Build history of the part. All positions in model axes, mm. Face numbers are marked on the shaded views. A direction names the side the tool comes from. Coordinates: 2 decimals unless noted, no trailing zeros. Order: outer loops, then holes, each group sorted by start corner. A loop starts at its lowest first (then second) coordinate and runs counter-clockwise, first axis right, second up. Notation, with made-up numbers: M -12.5,6.25 L 2.5,6.25 A19 ccw 2.5,30.25 Z; hole C 37,-18.5 d3. An arc over 180 degrees is marked long. Use a Markdown table: item, result. Add a question column.
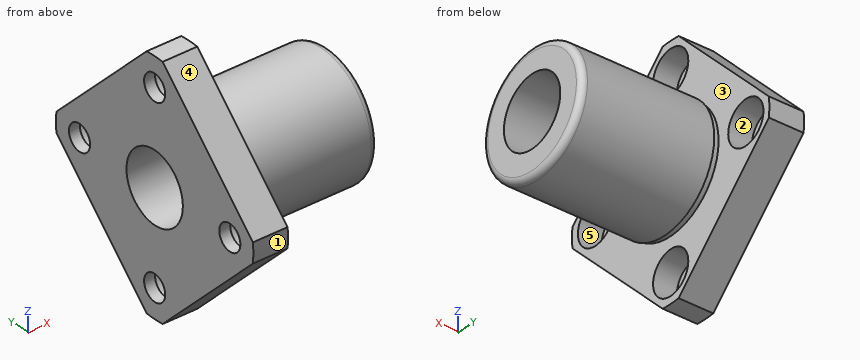
from build123d import *

# Parameters (mm, degrees)
BOSS_EXTRUDE1_DEPTH                              = 6
CBORE_FOR_M4_HEX_HEAD_MACHINE_SCREW1_D           = 4.5
CBORE_FOR_M4_HEX_HEAD_MACHINE_SCREW1_DEPTH       = 6
CBORE_FOR_M4_HEX_HEAD_MACHINE_SCREW1_CBORE_D     = 7.5
CBORE_FOR_M4_HEX_HEAD_MACHINE_SCREW1_CBORE_DEPTH = 4.1
F_12_0_12_DIAMETER_HOLE1_D                       = 12
F_12_0_12_DIAMETER_HOLE1_DEPTH                   = 30


with BuildPart() as part:
    # Sketch1 → Boss-Extrude1 (new body)
    with BuildSketch(Plane(origin=(0, 0, 0), x_dir=(0, -1, 0), z_dir=(-1, 0, 0))):
        with BuildLine():
            Line((-1.696016468, 20.93140053), (-20.93140053, 1.696016468))
            ThreePointArc((-20.93140053, 1.696016468), (-21, 0), (-20.93140053, -1.696016468))
            Line((-20.93140053, -1.696016468), (-1.696016468, -20.93140053))
            ThreePointArc((-1.696016468, -20.93140053), (0, -21), (1.696016468, -20.93140053))
            Line((1.696016468, -20.93140053), (20.93140053, -1.696016468))
            ThreePointArc((20.93140053, -1.696016468), (21, 0), (20.93140053, 1.696016468))
            Line((20.93140053, 1.696016468), (1.696016468, 20.93140053))
            ThreePointArc((1.696016468, 20.93140053), (0, 21), (-1.696016468, 20.93140053))
        make_face()
    extrude(amount=-BOSS_EXTRUDE1_DEPTH)

    # Sketch2 → Revolve1 (revolve)
    with BuildSketch(Plane(origin=(0, 0, 0), x_dir=(-1, 0, 0), z_dir=(0, 0, -1))):
        with BuildLine():
            Line((-30, 9.45), (-30, 0))
            Line((-30, 0), (-6, 0))
            Line((-6, 0), (-6, 10.2))
            Line((-6, 10.2), (-7, 10.2))
            Line((-7, 10.2), (-7, 10.5))
            Line((-7, 10.5), (-28.95, 10.5))
            ThreePointArc((-28.95, 10.5), (-29.69246212, 10.19246212), (-30, 9.45))
        make_face()
    revolve(axis=Axis((30.00125, 0, 0), (-1, 0, 0)))

    # CBORE for M4 Hex Head Machine Screw1
    with Locations(Plane(origin=(6, 0, 0), x_dir=(0, 0, -1), z_dir=(1, 0, 0))):
        with Locations((0, -16), (16, 0), (-16, 0), (0, 16)):
            CounterBoreHole(CBORE_FOR_M4_HEX_HEAD_MACHINE_SCREW1_D / 2, CBORE_FOR_M4_HEX_HEAD_MACHINE_SCREW1_CBORE_D / 2, CBORE_FOR_M4_HEX_HEAD_MACHINE_SCREW1_CBORE_DEPTH, depth=CBORE_FOR_M4_HEX_HEAD_MACHINE_SCREW1_DEPTH)

    # Ø12.0 (12) Diameter Hole1
    with Locations(Plane(origin=(30, 0, 0), x_dir=(0, 0, -1), z_dir=(1, 0, 0))):
        with Locations((0, 0)):
            Hole(F_12_0_12_DIAMETER_HOLE1_D / 2, depth=F_12_0_12_DIAMETER_HOLE1_DEPTH)


solid = part.part
(1) Which spindle directions (+Z, -Z, +X, -X, +Y, -Y) get a long thin tool onto all of the face, cutting with end or side? Do the marked faces 4 and 5. Say none if no direction does.
(2) Mould opens along Y. For the marked faces 1, 2 and 3 say: released by +Y, released by -Y, zero draft, split by the parting line, or undercut.
(3) Slice it at C-C on y = -16. Give the cut face in (x, z), and give its area (3 significant figures).
(4) Drill centre lines: line 1 along X through (y, z) = (-2.5, 13.5); line 2 along X through (y, z) = (14, -5); line 3 along Z through (x, y) = (10, -2). Where is each one in solid material? Low to high. Write a range as from..to.
(5) Drop flat-ended pins along their axis: P1, Ø2, axis at y = 17, z = 0.5, coming from the +X side; P2, Ø6, axis at y = -0.5, z = 14.5, coming from the +X side; P3, Ø6, axis at x = 24.5, z = 4, coming from the +Y side; P4, Ø5, axis at x = 19, z = 8, coming from the +Y side. Give the stop position or say it passes through.
(6) Slice it at D-D on z = -16.5. Give the cut face in (x, y), and give its area (3 significant figures).
(7) Slice it at A-A on z = 0. State how many separate pieces and enclosed holes the cut face has, and give its area (3 significant figures).
Solutions:
| question | item | result |
|---|---|---|
| 1 | face 4 | +Z, +X, -X, -Y |
| 1 | face 5 | +X |
| 2 | face 1 | released by -Y |
| 2 | face 2 | undercut |
| 2 | face 3 | zero draft |
| 3 | outline | M 0,-6.63 L 6,-6.63 L 6,-3.75 L 1.9,-3.75 L 1.9,-2.25 L 0,-2.25 Z; M 0,2.25 L 1.9,2.25 L 1.9,3.75 L 6,3.75 L 6,6.63 L 0,6.63 Z |
| 3 | area | 40.2 mm² |
| 4 | line 1 | 0..1.9 |
| 4 | line 2 | 0..6 |
| 4 | line 3 | -10.31..-5.66, 5.66..10.31 |
| 5 | P1 | through |
| 5 | P2 | x = 6 |
| 5 | P3 | y = 10.45 |
| 5 | P4 | y = 8.94 |
| 6 | outline | M 0,-6.13 L 6,-6.13 L 6,-3.72 L 1.9,-3.72 L 1.9,-2.19 L 0,-2.19 Z; M 0,2.19 L 1.9,2.19 L 1.9,3.72 L 6,3.72 L 6,6.13 L 0,6.13 Z |
| 6 | area | 34.7 mm² |
| 7 | separate pieces | 4 |
| 7 | enclosed holes | 0 |
| 7 | area | 316 mm² |
